For this review, take the finished solid that the model builds, in its own axes (mm). A direction names the side the tool comes from. Give positions to 0.01 mm unless a question says otherwise; leave off trailing zeros. Order: outer loops, then holes, each group sorted by start corner. A loop starts at its lowest first (then second) coordinate and runs counter-clockwise, first axis right, second up. Notation, with made-up numbers: (60.25, -1) -> (92.25, -1) arc R30 cw to (92.25, 33) -> close; hole circle Ø3 at (65.5, 75.5). An arc over 180 degrees is marked (long way). Use CSV: the item, a comma, the result in double quotes. Start each with the question number.
```python
from build123d import *

# Parameters (mm, degrees)
BOSS_EXTRUDE1_DEPTH = 17
CUT_EXTRUDE1_DEPTH  = 31
SKETCH3_W           = 9.47
SKETCH3_H           = 10.75
CUT_EXTRUDE2_REACH  = 41.287
SKETCH6_W           = 10
SKETCH6_H           = 10.75
SKETCH7_R           = 4
CUT_EXTRUDE3_DEPTH  = 31


with BuildPart() as part:
    # Sketch1 → Boss-Extrude1 (new body)
    with BuildSketch(Plane.XY):
        Polygon((0, 0), (0, 11.1), (5.04, 11.1), (5.04, -3.9), (-1.16650456, -19.86), (-6.626200647, -23.639063196), (-23.319289693, -8.973826134), (-26.37555014, -4.558379149), (-26.37555014, 11.1), (-21.33555014, 11.1), (-21.33555014, 0), align=None)
    extrude(amount=BOSS_EXTRUDE1_DEPTH)

    # Sketch2 → Cut-Extrude1 (cut, symmetric)
    with BuildSketch(Plane.ZY):
        Polygon((8.228054067, 11.1), (17, 11.1), (17, 12.88110255), (0, 12.88110255), (0, 11.1), align=None)
        with BuildLine():
            ThreePointArc((0, 0), (2.28131811, 6.908525055), (8.228054067, 11.1))
            Line((8.228054067, 11.1), (0, 11.1))
            Line((0, 11.1), (0, 0))
        make_face()
        Polygon((13.228054067, 10.512247596), (17, 6.76), (17, 11.1), (8.228054067, 11.1), align=None)
    extrude(amount=CUT_EXTRUDE1_DEPTH, both=True, mode=Mode.SUBTRACT)

    # Cut-Sweep1: sweep along a path in Sketch5
    with BuildLine(Plane.XY.offset(7)) as cut_sweep1_path:
        Line((-11.079626433, -19.726633046), (-3.773757644, -14.201247879))
    # Sketch3 → Cut-Sweep1 (sweep, cut)
    with BuildSketch(Plane(origin=(-14.60747623, -16.627341271, 0), x_dir=(-0.7512641335035073, 0.6600016679609412, 0), z_dir=(-0.6600016679609412, -0.7512641335035074, 0))):
        with Locations((-1.868794251, -9.115)):
            Rectangle(SKETCH3_W, SKETCH3_H)
    sweep(path=cut_sweep1_path.line, mode=Mode.SUBTRACT)

    # Cut-Extrude2: up to this face of the body (flat: up to its plane)
    cut_extrude2_end = Plane(part.part.faces().sort_by_distance((-5.99334807, -18.223163907, 9.115))[0])
    # Sketch6 → Cut-Extrude2 (cut, up to the picked face)
    with BuildSketch(Plane(origin=(0, 0, 0), x_dir=(1, 0, 0), z_dir=(0, 1, 0)), mode=Mode.PRIVATE) as cut_extrude2_sk1:
        with Locations((-8.42, -9.115)):
            Rectangle(SKETCH6_W, SKETCH6_H)
    cut_extrude2_tool1 = split(extrude(cut_extrude2_sk1.sketch, amount=-CUT_EXTRUDE2_REACH, mode=Mode.PRIVATE), bisect_by=cut_extrude2_end, keep=Keep.BOTH, mode=Mode.PRIVATE)
    add(cut_extrude2_tool1.solids().sort_by(Axis((-8.42, 0, 9.115), (0, -1, 0)))[0], mode=Mode.SUBTRACT)

    # Sketch7 → Cut-Extrude3 (cut, symmetric)
    with BuildSketch(Plane.ZY.offset(10.66777507)):
        with Locations(Location((8.5, 4.041620851, 0), (0, 0, 270))):
            Circle(SKETCH7_R)
    extrude(amount=CUT_EXTRUDE3_DEPTH, both=True, mode=Mode.SUBTRACT)


solid = part.part
```
1. Clearance check with flat-ended pins moving along their axes: P1, Ø6.5, axis at y = 4.04, z = 8.5, coming from the +X side; P2, Ø5, axis at x = -15.5, z = 7.5, coming from the +Y side; P3, Ø1.5, axis at y = -11, z = 13, coming from the +X side; P4, Ø1, axis at x = -21.5, z = 12, coming from the -Y side. State where each tip first meets the part, or that it passes through.
2. Consider section C-C (z = 9.75). State the section outline as (x, y) points, plus the area to 3 significant figures.
3. Draft analysis for pull direction Z (two halves, no side actions). For faces 6 (the face through (-23.891, 4.909, 4.595)), 7 (the face through (1.98, -11.77, 8.38)), 8 (the face through (-15.067, -13.455, 9.19)), 9 (the face through (2.5, 6.8, 2.2)), state which applies: +Z half, -Z half, draft (parallel to the pull), parting line (faces both ways), or undercut.
4. To check wall thickness, follow L1, parallel to Z at x = -8.5, y = -9; L2, parallel to X at y = -2, z = 10.5; L3, parallel to X at y = 10.5, z = 9.75. State the ranges of each line that lie inside material, in increasing order. Write a range as [from, to].
5. Consider section D-D (x = -22.5). State the section outline as (y, z) points, plus the area to 3 significant figures.
6. Consider section B-B (y = 3). State the section outline as (x, z) points, plus the area to 3 significant figures.
7. Consider section A-A (y = -2). State the section outline as (x, z) points.
8. For faces 1 (the face through (-21.336, 8, 10)), 2 (the face through (-23.9, 6.8, 2.2)), 3 (the face through (-3.42, -7, 9)), 4 (the face through (-13.42, -6, 9)), 5 (the face through (-3.858, -21.723, 8.381)), list the 3-axis set-ups (+Z, -Z, +X, -X, +Y, -Y) from which the entire face can be reached by the end or side of a thin tool; tool diameter is ignored.
Answer list:
1,P1,"through"
1,P2,"y = 0"
1,P3,"x = 2.57"
1,P4,"y = -11.01"
2,outline,"(-26.38, -4.56) -> (-23.32, -8.97) -> (-16.76, -14.74) -> (-13.42, -12.21) -> (-13.42, 0) -> (-21.34, 0) -> (-21.34, 0.24) -> (-26.38, 0.24) -> close; (-26.38, 7.84) -> (-21.34, 7.84) -> (-21.34, 10.92) -> (-26.38, 10.92) -> close; (-9.65, -20.99) -> (-6.63, -23.64) -> (-1.17, -19.86) -> (5.04, -3.9) -> (5.04, 0.24) -> (0, 0.24) -> (0, 0) -> (-3.42, 0) -> (-3.42, -14.51) -> (-2.34, -15.46) -> close; (0, 7.84) -> (5.04, 7.84) -> (5.04, 10.92) -> (0, 10.92) -> close"
2,area,"320 mm2"
3,face 6,"undercut"
3,face 7,"draft"
3,face 8,"undercut"
3,face 9,"-Z half"
4,L1,"[0, 3.74], [14.49, 17]"
4,L2,"[-26.38, -13.42], [-3.42, 5.04]"
4,L3,"[-26.38, -21.34], [0, 5.04]"
5,outline,"(-9.69, 0) -> (0, 0) arc R11.6 ccw to (11.1, 8.23) -> (10.51, 13.23) -> (6.76, 17) -> (-9.69, 17) -> close; hole circle Ø8 at (4.04, 8.5)"
5,area,"268 mm2"
6,outline,"(-26.38, 0.39) -> (-21.34, 0.39) -> (-21.34, 4.64) -> (-26.38, 4.64) -> close; (-26.38, 12.36) -> (-21.34, 12.36) -> (-21.34, 17) -> (-26.38, 17) -> close; (0, 0.39) -> (5.04, 0.39) -> (5.04, 4.64) -> (0, 4.64) -> close; (0, 12.36) -> (5.04, 12.36) -> (5.04, 17) -> (0, 17) -> close"
6,area,"89.5 mm2"
7,outline,"(-26.38, 0) -> (5.04, 0) -> (5.04, 17) -> (-26.38, 17) -> close; hole (-13.42, 3.74) -> (-3.42, 3.74) -> (-3.42, 14.49) -> (-13.42, 14.49) -> close"
8,face 1,"+Z, -Z, +Y"
8,face 2,"-Z, +X, -X, +Y"
8,face 3,"+Y"
8,face 4,"+Y, -Y"
8,face 5,"+Z, -Z, +X, -Y"
